Can you work these out from the drawing? Everything is in mm from the part's minimum corner. Coordinates: 2 decimals unless noted, no trailing zeros. Loops run counter-clockwise (first coordinate to the right, second up) from the corner with the lowest first, then second, coordinate; pieces in that order, holes last.
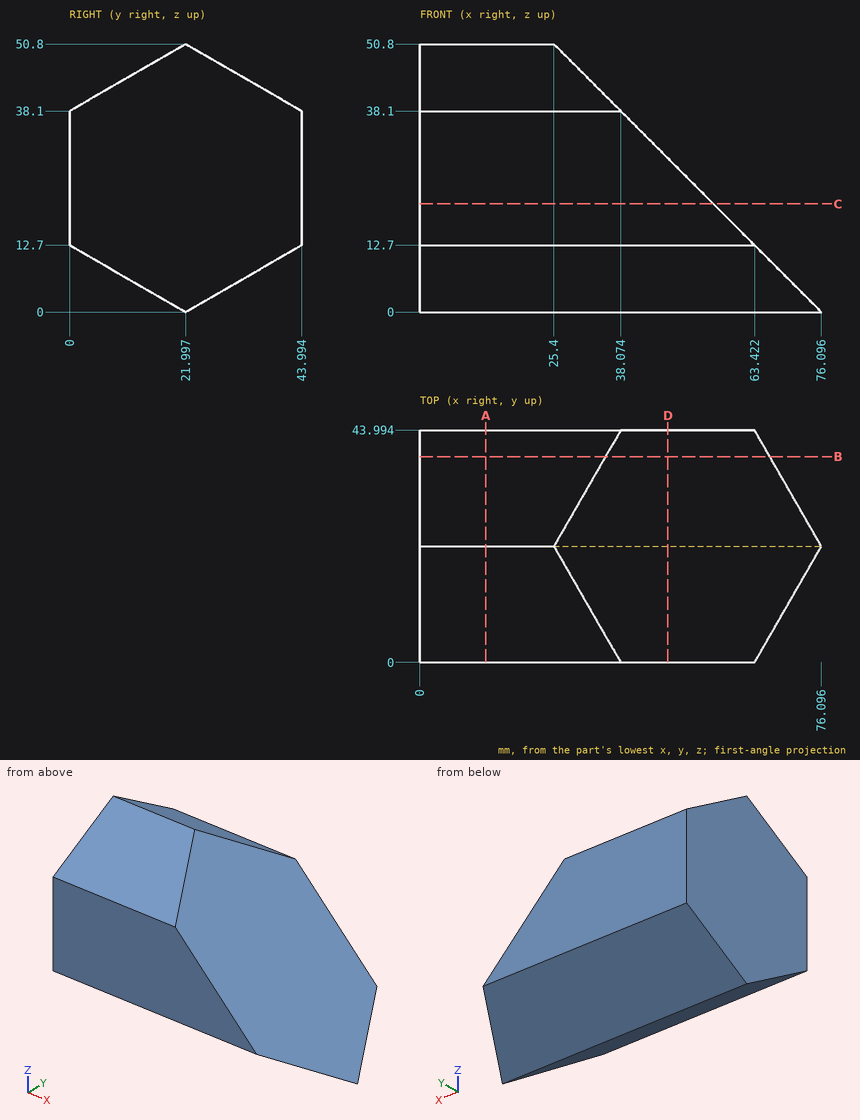
1. I want a section at C-C (z = 20.5). Please give me the cut outline in (x, y), then the cut area to 3 significant figures.
2. I need wall thicknesses on line 1 along Z through (x, y) = (23, 42); line 2 along X through (y, z) = (38.5, 29.5) (1 decimal); line 3 along X through (y, z) = (36.5, 34.5) (1 decimal). Which ranges of each line are inside material? Lowest first, please.
3. I want a section at A-A (x = 12.5). Please give me the cut outline in (y, z), then the cut area to 3 significant figures.
4. I want a section at D-D (x = 47). Please give me the cut outline in (y, z), then the cut area to 3 significant figures.
5. For pin 1 (6 mm diameter, centred on x = 31, y = 28, fed in from -Z); pin 2 (5 mm diameter, centred on x = 32.5, y = 37.5, fed in from +Z); pin 3 (5 mm diameter, centred on x = 57.5, y = 31, fed in from +Z), each with a flat end and sliding along its axis, tell me the tip position at first contact or that it passes through.
6. I want a section at B-B (y = 39). Please give me the cut outline in (x, z), then the cut area to 3 significant figures.
Response values:
1. outline: (0, 0) - (55.64, 0) - (55.64, 43.99) - (0, 43.99) - close
1. area: 2,450 mm2
2. line 1: z = 11.55 to 39.25
2. line 2: x = 0 to 46.7
2. line 3: x = 0 to 41.7
3. outline: (0, 12.7) - (22, 0) - (43.99, 12.7) - (43.99, 38.1) - (22, 50.8) - (0, 38.1) - close
3. area: 1,680 mm2
4. outline: (0, 12.7) - (22, 0) - (43.99, 12.7) - (43.99, 29.16) - (0, 29.16) - close
4. area: 1,000 mm2
5. pin 1: stops at z = 1.73
5. pin 2: stops at z = 43.29
5. pin 3: stops at z = 21.14
6. outline: (0, 9.82) - (66.3, 9.82) - (35.2, 40.98) - (0, 40.98) - close
6. area: 1,580 mm2
